Read the model definition and answer for the solid it produces. Units are mm, in the model's axes. Face numbers are marked on the shaded views. A direction names the side the tool comes from. Round coordinates to 2 decimals unless told otherwise and drop trailing zeros. Write each loop counter-clockwise with the first axis right and the second up, starting at its lowest first coordinate (ties: lowest second). Pieces come first, ordered by that corner, then holes. Notation, with made-up numbers: (87.5, 32.5) - (110.5, 32.5) arc R26 ccw to (110.5, 48.5) - close; hole circle Ø9 at (-32.5, 61.25). An arc over 180 degrees is marked (long way). Use one line per item in the form item = value. Start each with the question number.
1) The part is cut by section B-B, the plane z = 5. Give the vertices of the cut face in (x, y), plus the area to 3 significant figures.
2) For the marked faces 1, 2 and 3, determine the directions among +Z, -Z, +X, -X, +Y, -Y from which every point of the face is accessible in a straight line to the end or side of a thin tool.
3) The part is cut by section D-D, the plane y = -16.5. Give the vertices of the cut face in (x, z).
4) Each of these flat-tipped pins is pushed along its axis until it touches: pin 1 (8 mm diameter, centred on y = -5, z = 17.5, fed in from -X); pin 2 (5 mm diameter, centred on x = -4, z = 4.5, fed in from -Y); pin 3 (8 mm diameter, centred on x = -3.5, z = 22, fed in from -Y); pin 4 (19 mm diameter, centred on x = 0, y = 0, fed in from -Z). Where does it stop, or does it pass through?
5) The part is cut by section C-C, the plane x = 0. Give the vertices of the cut face in (y, z), plus the area to 3 significant figures.
6) For a pull along X with two mould halves and no side action, classify the marked faces 4, 5 and 6 as released by +X, released by -X, zero draft, split by the parting line, or undercut.
7) Consider line 1 along X through (y, z) = (0, 27.5); line 2 along Z through (x, y) = (-5, 8). Determine where each line is inside the solid, lowest interval first. Write a range as from..to.
8) The part is cut by section A-A, the plane y = 2.5. Give the vertices of the cut face in (x, z).
Autodesk Inventor part; units mm, degrees
ref_plane "Work Plane7" through (-38, -38, 25) normal (0, 0, -1) x (0, 1, 0)
ref_plane "YZ Plane" through (0, 0, 0) normal (1, 0, 0) x (0, 1, 0)
ref_plane "XZ Plane" through (0, 0, 0) normal (0, 1, 0) x (-1, 0, 0)
sketch "Sketch1" plane through (0, 0, 0) normal (0, 0, 1) x (1, 0, 0)
  circle A0 centre (0, 0) radius 27.5
  circle A1 centre (0, 0) radius 35
  line L0 (16, 0) -> (-8, -13.8564)
  line L1 (-8, 13.8564) -> (16, 0)
  line L2 (-8, -13.8564) -> (-8, 13.8564)
  circle A2 centre (0, 0) radius 25
  circle A3 centre (-25, 0) radius 5
  circle A4 centre (-21.6506, 12.5) radius 5
  circle A5 centre (-12.5, 21.6506) radius 5
  circle A6 centre (0, 25) radius 5
  circle A7 centre (0, 0) radius 38
  point P0 (4.9749, 24.5)
  point P1 (-4.9749, 24.5)
  point P2 (-7.9416, 23.7051)
  point P3 (-16.5584, 18.7302)
  point P4 (-18.7302, 16.5584)
  point P5 (-23.7051, 7.9416)
  point P6 (-24.5, 4.9749)
  point P7 (-24.5, -4.9749)
  dimension "d5" = 70
  dimension "d14" = 10
  dimension "d15" = 10
  dimension "d18" = 90
ref_plane "Work Plane7" through (-38, -38, 25) normal (0, 0, -1) x (0, 1, 0)
extrude "Extrusion1" add sketch "Sketch1" along normal up to surface (25 mm away) contours A3 A2 A4 A5 A6
fillet "Fillet1" radius 2 6 edges at (-24.5, 4.9749, 12.5) (-23.7051, 7.9416, 12.5) (-18.7302, 16.5584, 12.5) (-16.5584, 18.7302, 12.5) (-7.9416, 23.7051, 12.5) (-4.9749, 24.5, 12.5)
sketch "Sketch3" plane through (0, 0, 25) normal (0, 0, 1) x (0, 1, 0)
  circle A0 centre (0, 0) radius 28
  circle A1 centre (0, 0) radius 6
  circle A2 centre (0, 0) radius 27.5
  dimension "d13" = 0.5
extrude "Extrusion3" add sketch "Sketch3" along normal blind 10 contours A2
properties part number "handle_base2"
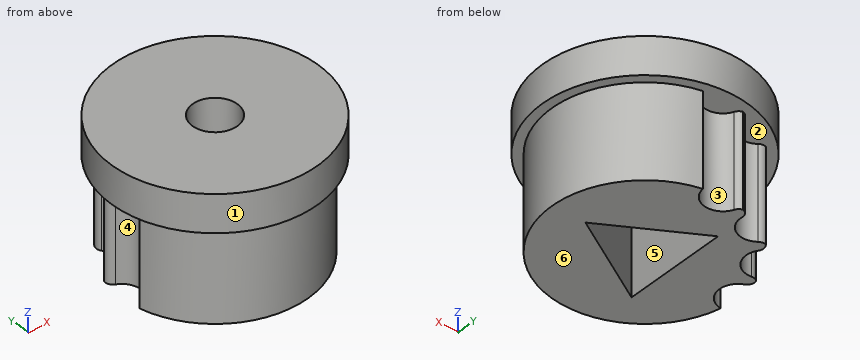
Geometry results:
q1.outline = (-24.5, -4.97) arc R25 ccw (long way) to (4.97, 24.5) arc R5 cw to (-4.62, 23.08) arc R2 ccw to (-6.01, 24.27) arc R2 ccw to (-7.52, 22.13) arc R5 cw to (-15.54, 17.68) arc R2 ccw to (-17.34, 18.01) arc R2 ccw to (-17.58, 15.41) arc R5 cw to (-22.3, 7.54) arc R2 ccw to (-24.02, 6.93) arc R2 ccw to (-22.93, 4.55) arc R5 cw to start; hole (-8, -13.86) - (16, 0) - (-8, 13.86) - close
q1.area = 1,480 mm2
q2.face_1 = +Z, -Z
q2.face_2 = -Z
q2.face_3 = -Z, +Y
q3.outline = (-22, 25) - (-18.78, 25) - (-18.78, 0) - (18.78, 0) - (18.78, 25) - (22, 25) - (22, 35) - (-22, 35) - close
q4.pin_1 = -24.5
q4.pin_2 = -24.95
q4.pin_3 = -27.49
q4.pin_4 = 0
q5.outline = (-27.5, 25) - (-25, 25) - (-25, 0) - (-9.24, 0) - (-9.24, 25) - (-6, 25) - (-6, 35) - (-27.5, 35) - close; (6, 25) - (9.24, 25) - (9.24, 0) - (20, 0) - (20, 25) - (27.5, 25) - (27.5, 35) - (6, 35) - close
q5.area = 1,090 mm2
q6.face_4 = released by -X
q6.face_5 = undercut
q6.face_6 = zero draft
q7.line_1 = -27.5..-6, 6..27.5
q7.line_2 = 25..35
q8.outline = (-27.39, 25) - (-20.67, 25) - (-20.67, 0) - (-8, 0) - (-8, 25) - (-5.45, 25) - (-5.45, 35) - (-27.39, 35) - close; (5.45, 25) - (11.67, 25) - (11.67, 0) - (24.87, 0) - (24.87, 25) - (27.39, 25) - (27.39, 35) - (5.45, 35) - close
